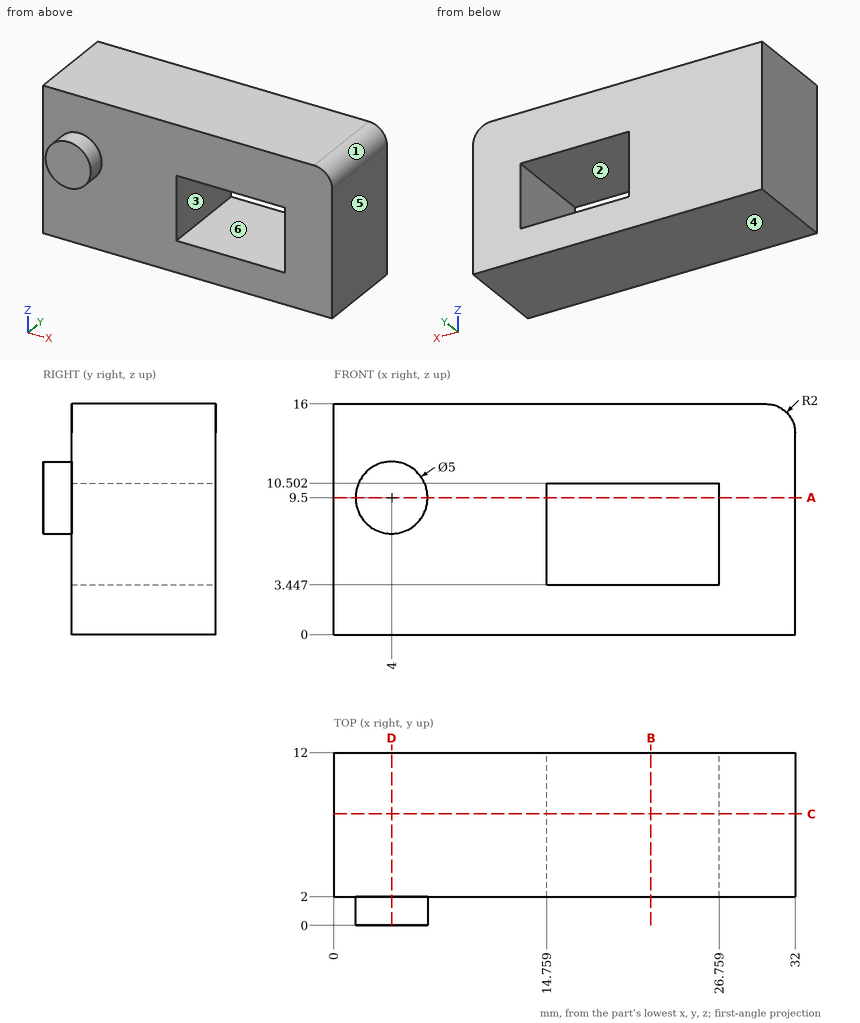
Print and shaded views of the part. All mm, measured from the part's lowest x, y and z. A direction names the side the tool comes from. Round coordinates to 2 decimals unless told otherwise and drop trailing zeros. Write each loop counter-clockwise with the first axis right and the second up, starting at its lowest first coordinate (ties: lowest second). Pieces come first, ordered by that corner, then holes. Notation, with made-up numbers: M 39,17.25 L 89,17.25 A31 cw 89,51.25 Z; hole C -17.75,8.25 d7. An arc over 180 degrees is marked long. One line per question, with ' | ' between items.
(1) Probe line 1 along Z through (x, y) = (20, 4.75); line 2 along X through (y, z) = (6, 6.5); line 3 along Y through (x, z) = (7, 10.25). List the from-to ranges inside material, lowest first.
Answer key:
line 1: z = 0 to 3.45, 10.5 to 16 | line 2: x = 0 to 14.76, 26.76 to 32 | line 3: y = 2 to 12
(2) Saw through at A-A on z = 9.5. Write the cut outline in (x, y).
Answer key:
outline: M 0,2 L 1.5,2 L 1.5,0 L 6.5,0 L 6.5,2 L 14.76,2 L 14.76,12 L 0,12 Z; M 26.76,2 L 32,2 L 32,12 L 26.76,12 Z
(3) 3-axis set-ups, long thin cutter, end or side, ignore diameter. For the marked faces 1 and 2: which of +Z, -Z, +X, -X, +Y, -Y reach the whole face in a straight line?
Answer key:
face 1: +Z, +X, +Y, -Y | face 2: +Y, -Y
(4) Two-plate mould, pull along X, no slides. Class the marked faces 3, 4, 5 and 6: released by +X, released by -X, zero draft, split by the parting line, or undercut.
Answer key:
face 3: undercut | face 4: zero draft | face 5: released by +X | face 6: undercut
(5) Pin check, flat tip, straight feed: pin 1 (1 mm diameter, centred on x = 25.5, z = 14, fed in from -Y). Stop position of the tip, or through.
Answer key:
pin 1: stops at y = 2
(6) Saw through at D-D on x = 4. Write the cut outline in (y, z).
Answer key:
outline: M 0,7 L 2,7 L 2,0 L 12,0 L 12,16 L 2,16 L 2,12 L 0,12 Z
(7) Saw through at C-C on y = 7.75. Write the cut outline in (x, z).
Answer key:
outline: M 0,0 L 32,0 L 32,14 A2 ccw 30,16 L 0,16 Z; hole M 14.76,3.45 L 26.76,3.45 L 26.76,10.5 L 14.76,10.5 Z
(8) Saw through at B-B on x = 22. Write the cut outline in (y, z).
Answer key:
outline: M 2,0 L 12,0 L 12,3.45 L 2,3.45 Z; M 2,10.5 L 12,10.5 L 12,16 L 2,16 Z
